```python
from build123d import *

# Parameters (mm, degrees)
SKETCH1_W           = 25.4
SKETCH1_H           = 50.8
SKETCH1_W_2         = 20.32
SKETCH1_H_2         = 45.72
EXTRUDE_THIN1_DEPTH = 69.85
SKETCH2_R           = 3.175
CUT_EXTRUDE1_DEPTH  = 26.4
SKETCH4_R           = 2.4765
CUT_EXTRUDE3_DEPTH  = 51.8


with BuildPart() as part:
    # Sketch1 → Extrude-Thin1 (new body, symmetric)
    with BuildSketch(Plane.XY):
        Rectangle(SKETCH1_W, SKETCH1_H)
        Rectangle(SKETCH1_W_2, SKETCH1_H_2, mode=Mode.SUBTRACT)
    extrude(amount=EXTRUDE_THIN1_DEPTH, both=True)

    # Sketch2 → Cut-Extrude1 (cut, through all)
    with BuildSketch(Plane(origin=(12.7, 0, 0), x_dir=(0, 0, -1), z_dir=(1, 0, 0))):
        with Locations((55.7022, 0)):
            Circle(SKETCH2_R)
    extrude(amount=-CUT_EXTRUDE1_DEPTH, mode=Mode.SUBTRACT)

    # Sketch4 → Cut-Extrude3 (cut, through all)
    with BuildSketch(Plane(origin=(0, 25.4, 0), x_dir=(1, 0, 0), z_dir=(0, 1, 0))):
        with Locations((0, -57.15)):
            Circle(SKETCH4_R)
    extrude(amount=-CUT_EXTRUDE3_DEPTH, mode=Mode.SUBTRACT)


solid = part.part
```
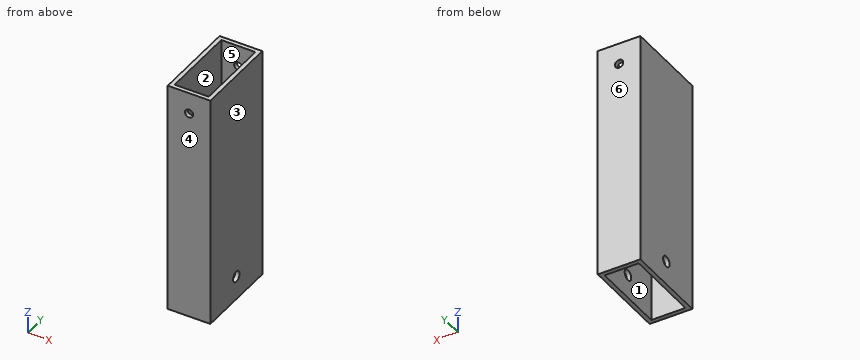
Source: CAD feature listing. Evaluate the final solid. Frame: model axes, mm. Face numbers are marked on the shaded views. A direction names the side the tool comes from. Round coordinates to 2 decimals unless told otherwise and drop trailing zeros. Loops run counter-clockwise (first coordinate to the right, second up) from the corner with the lowest first, then second, coordinate; pieces in that order, holes last. Notation, with made-up numbers: M -1.75,-5 L 31.25,-5 A15 cw 31.25,3 Z; hole C 22,-30.5 d2. An arc over 180 degrees is marked long. Use a Markdown table: item, result. Add a question column.
1. Set-up query: the marked faces 5 and 6. Return all of +Z, -Z, +X, -X, +Y, -Y with unobstructed straight access to the full face (end or side cutting, diameter ignored); none if empty.
2. Cut plane C-C, the plane z = 57.15. Output: boundary loops of the cut face in (x, y).
3. Pull-direction query (X, two-part tool) for the marked faces 1, 2, 3 and 4; classes: +X half, -X half, draft (parallel to the pull), parting line (faces both ways), or undercut.
4. Cut plane D-D, the plane x = 0. Output: boundary loops of the cut face in (y, z).
5. Cut plane B-B, the plane z = -13. Output: boundary loops of the cut face in (x, y).
6. Ray query, line 1 along X through (y, z) = (3.5, 23); line 2 along Y through (x, z) = (1.25, -58); line 3 along Z through (x, y) = (0, -23.7). Return the intervals inside material, ascending. Write a range as [from, to].
7. Cut plane A-A, the plane y = 0. Output: boundary loops of the cut face in (x, z).
Solution:
| question | item | result |
|---|---|---|
| 1 | face 5 | +Z, -Z |
| 1 | face 6 | +Z, -Z, +X, -X, +Y |
| 2 | outline | M -12.7,-25.4 L -2.48,-25.4 L -2.48,-22.86 L -10.16,-22.86 L -10.16,22.86 L -2.48,22.86 L -2.48,25.4 L -12.7,25.4 Z; M 2.48,-25.4 L 12.7,-25.4 L 12.7,25.4 L 2.48,25.4 L 2.48,22.86 L 10.16,22.86 L 10.16,-22.86 L 2.48,-22.86 Z |
| 3 | face 1 | undercut |
| 3 | face 2 | undercut |
| 3 | face 3 | +X half |
| 3 | face 4 | draft |
| 4 | outline | M -25.4,-69.85 L -22.86,-69.85 L -22.86,54.67 L -25.4,54.67 Z; M -25.4,59.63 L -22.86,59.63 L -22.86,69.85 L -25.4,69.85 Z; M 22.86,-69.85 L 25.4,-69.85 L 25.4,54.67 L 22.86,54.67 Z; M 22.86,59.63 L 25.4,59.63 L 25.4,69.85 L 22.86,69.85 Z |
| 5 | outline | M -12.7,-25.4 L 12.7,-25.4 L 12.7,25.4 L -12.7,25.4 Z; hole M -10.16,-22.86 L 10.16,-22.86 L 10.16,22.86 L -10.16,22.86 Z |
| 6 | line 1 | x = [-12.7, -10.16], [10.16, 12.7] |
| 6 | line 2 | y = [-25.4, -22.86], [22.86, 25.4] |
| 6 | line 3 | z = [-69.85, 54.67], [59.63, 69.85] |
| 7 | outline | M -12.7,-69.85 L -10.16,-69.85 L -10.16,-58.88 L -12.7,-58.88 Z; M -12.7,-52.53 L -10.16,-52.53 L -10.16,69.85 L -12.7,69.85 Z; M 10.16,-69.85 L 12.7,-69.85 L 12.7,-58.88 L 10.16,-58.88 Z; M 10.16,-52.53 L 12.7,-52.53 L 12.7,69.85 L 10.16,69.85 Z |
